Geometry check sheet. Reference: the model listing, model coordinates, mm. A direction names the side the tool comes from. Coordinates: 2 decimals unless noted, no trailing zeros. Write each loop counter-clockwise with the first axis right and the second up, starting at its lowest first coordinate (ties: lowest second). Pieces come first, ordered by that corner, then holes. Notation, with made-up numbers: (-13, 4) -> (29, 4) arc R9 ccw to (29, 13) -> close; hole circle Ø4 at (51.25, 41.25). An arc over 180 degrees is marked (long way). Use a Markdown table: item, result.
Autodesk Inventor part; units mm, degrees
ref_plane "Start plane" through (0, 0, 0) normal (0, 0, 1) x (1, 0, 0)
ref_plane "End plane" through (0, 0, 560) normal (0, 0, 1) x (1, 0, 0)
ref_plane "Work Plane4" through (0, -20, 0) normal (0, 0.7071, -0.7071) x (1, 0, 0)
ref_plane "Start plane" through (0, 0, 0) normal (0, 0, 1) x (1, 0, 0)
ref_plane "End plane" through (0, 0, 560) normal (0, 0, 1) x (1, 0, 0)
sketch "Sketch" plane through (0, 0, 0) normal (0, 0, 1) x (1, 0, 0)
  line L0 (-20, -13.4) -> (-20, 13.4)
  line L1 (-13.4, 20) -> (13.4, 20)
  line L2 (20, 13.4) -> (20, -13.4)
  line L3 (13.4, -20) -> (-13.4, -20)
  arc A0 (-20, -13.4) -> (-13.4, -20) centre (-13.4, -13.4) ccw
  arc A1 (-13.4, 20) -> (-20, 13.4) centre (-13.4, 13.4) ccw
  arc A2 (20, 13.4) -> (13.4, 20) centre (13.4, 13.4) ccw
  arc A3 (13.4, -20) -> (20, -13.4) centre (13.4, -13.4) ccw
  arc A4 (-13.4, 17) -> (-17, 13.4) centre (-13.4, 13.4) ccw
  line L4 (-13.4, 17) -> (13.4, 17)
  arc A5 (17, 13.4) -> (13.4, 17) centre (13.4, 13.4) ccw
  line L5 (17, 13.4) -> (17, -13.4)
  arc A6 (13.4, -17) -> (17, -13.4) centre (13.4, -13.4) ccw
  line L6 (13.4, -17) -> (-13.4, -17)
  arc A7 (-17, -13.4) -> (-13.4, -17) centre (-13.4, -13.4) ccw
  line L7 (-17, -13.4) -> (-17, 13.4)
  line L8 (0, 29.9137) -> (0, -29.9137) construction
  line L9 (-29.9137, 0) -> (29.9137, 0) construction
  dimension "d7" = 6.6
  dimension "d10" = 40
  dimension "d11" = 40
  dimension "d12" = 3
  dimension "d15" = 20
  dimension "d16" = 20
extrude "Body" add sketch "Sketch" along normal up to surface (560 mm away) from surface at 0
sketch "Sketch3" plane through (0, 0, 0) normal (0, 0, 1) x (1, 0, 0)
  line L0 (0, 0) -> (10, 0)
ref_plane "Work Plane3" through (0, 0, 0) normal (0, -1, 0) x (1, 0, 0)
sketch "Sketch4" plane through (0, 0, 0) normal (0, -1, 0) x (1, 0, 0)
  line L0 (-2, 0) -> (12, 0)
  line L1 (-2, 560) -> (12, 560)
  dimension "d18" = 560
ref_plane "Work Plane4" through (0, -20, 0) normal (0, 0.7071, -0.7071) x (1, 0, 0)
split "Split1" plane through (0, -20, 0) removes the side toward (0, 0.7071, -0.7071)
ref_plane "Work Plane5" through (1302, 597.6, 560) normal (0, 0, 1) x (1, 0, 0)
split "Split2" plane through (1302, 597.6, 560) removes the side toward (0, 0, 1)
equation "\"d7\" = G_IR"
equation "\"d10\" = G_H"
equation "\"d11\" = G_W"
equation "\"d12\" = G_T"
equation "\"d15\" = 0.5 * d10"
equation "\"d16\" = 0.5 * d11"
equation "\"d3\" = G_L"
equation "\"G_W\" = 40"
equation "\"G_H\" = 40"
equation "\"G_T\" = 3"
equation "\"G_IR\" = 6.6"
equation "\"G_L\" = d18"
equation "\"G_OFFSET_START\" = 0"
properties part number "DIN EN 10305-5 - 40 x 40 x 3  - 560" material "Steel, Mild"
Item 1: Depth check by flat-ended pin: P1, Ø1, axis at x = -15.5, z = 423.5, coming from the +Y side; P2, Ø5, axis at x = -14, z = 263.5, coming from the -Y side; P3, Ø12, axis at x = -4.5, y = 6.5, coming from the -Z side; P4, Ø5, axis at x = -14.5, y = 15, coming from the -Z side. Enter the tip coordinate at first touch or a pass-through.
Answer block:
| item | result |
|---|---|
| P1 | stops at y = 19.8 |
| P2 | stops at y = -20 |
| P3 | passes through |
| P4 | stops at z = 34.27 |
Item 2: Section check C-C on z = 108. Record the boundary of the cut face in (x, y).
Answer block:
| item | result |
|---|---|
| outline | (-20, -13.4) arc R6.6 ccw to (-13.4, -20) -> (13.4, -20) arc R6.6 ccw to (20, -13.4) -> (20, 13.4) arc R6.6 ccw to (13.4, 20) -> (-13.4, 20) arc R6.6 ccw to (-20, 13.4) -> close; hole (-17, -13.4) arc R3.6 ccw to (-13.4, -17) -> (13.4, -17) arc R3.6 ccw to (17, -13.4) -> (17, 13.4) arc R3.6 ccw to (13.4, 17) -> (-13.4, 17) arc R3.6 ccw to (-17, 13.4) -> close |
Item 3: Section check A-A on y = 8.5. Record the boundary of the cut face in (x, z), then the cut area to 3 significant figures.
Answer block:
| item | result |
|---|---|
| outline | (-20, 28.5) -> (-17, 28.5) -> (-17, 560) -> (-20, 560) -> close; (17, 28.5) -> (20, 28.5) -> (20, 560) -> (17, 560) -> close |
| area | 3,190 mm^2 |
Item 4: Tool access check on faces 1 (the flat face through (0, 17, 295)), 2 (the flat face through (20, 0, 279)). Record the directions out of +Z, -Z, +X, -X, +Y, -Y that give a thin tool (end or side, any length) a straight path to the whole face; none if there is none.
Answer block:
| item | result |
|---|---|
| face 1 | +Z, -Z |
| face 2 | +Z, -Z, +X, +Y, -Y |
Item 5: Section check B-B on x = -4. Record the boundary of the cut face in (y, z), then the cut area to 3 significant figures.
Answer block:
| item | result |
|---|---|
| outline | (-20, 0) -> (-17, 3) -> (-17, 560) -> (-20, 560) -> close; (17, 37) -> (20, 40) -> (20, 560) -> (17, 560) -> close |
| area | 3,240 mm^2 |
Item 6: Thickness scan on L1, parallel to X at y = -4.5, z = 61.5; L2, parallel to Y at x = 14, z = 488. Record the ranges inside material, lowest first. Write a range as [from, to].
Answer block:
| item | result |
|---|---|
| L1 | x = [-20, -17], [17, 20] |
| L2 | y = [-19.97, -16.95], [16.95, 19.97] |
Item 7: Mould release check, pull along Y, two halves, no side actions. Record for faces 3 (the flat face through (0, -20, 276)), 4 (the flat face through (17.5, 0.3, 20.3)), 5 (the flat face through (17, 0, 279)), 6 (the flat face through (-18, 0, 560)): +Y half, -Y half, draft (parallel to the pull), parting line (faces both ways), or undercut.
Answer block:
| item | result |
|---|---|
| face 3 | -Y half |
| face 4 | +Y half |
| face 5 | undercut |
| face 6 | draft |
